```python
from build123d import *

# Parameters (mm, degrees)
SALIENTE_EXTRUIR2_DEPTH      = 69
SALIENTE_EXTRUIR2_DEPTH_BACK = 69
CROQUIS3_R                   = 58
CROQUIS5_R                   = 58
CROQUIS5_R_2                 = 47.65301306
CROQUIS5_R_3                 = 3.895689101
SALIENTE_EXTRUIR3_DEPTH      = 2


with BuildPart() as part:
    # Croquis2 → Revolución1 (revolve)
    with BuildSketch(Plane.XY):
        Polygon((0, 0), (-58, 0), (-58, 68), (-42.5, 83.579391827), (-42.5, 378.579391827), (-58, 394.000404577), (-58, 462.000404577), (0, 462.000404577), align=None)
    revolve(axis=Axis((0, 462.000404577, 0), (0, -1, 0)))

    # Croquis3 → Saliente-Extruir2 (add, two sides: drawn at the far end of the back side and taken through both)
    with BuildSketch(Plane(origin=(0, 0, 0), x_dir=(0, 0, -1), z_dir=(1, 0, 0)).offset(-SALIENTE_EXTRUIR2_DEPTH_BACK)):
        with Locations((0, 462.000404577)):
            Circle(CROQUIS3_R)
        Circle(CROQUIS3_R)
    extrude(amount=SALIENTE_EXTRUIR2_DEPTH + SALIENTE_EXTRUIR2_DEPTH_BACK)

    # Croquis5 → Saliente-Extruir3 (add)
    # profile 1 of 2: a face of its own
    with BuildSketch(Plane(origin=(69, 0, 0), x_dir=(0, 0, -1), z_dir=(1, 0, 0))):
        Circle(CROQUIS5_R)
        Circle(CROQUIS5_R_2, mode=Mode.SUBTRACT)
        with Locations((0, 52.526315759)):
            Circle(CROQUIS5_R_3, mode=Mode.SUBTRACT)
        with Locations((49.95549488, 16.231524222)):
            Circle(CROQUIS5_R_3, mode=Mode.SUBTRACT)
        with Locations((30.874193761, -42.494682101)):
            Circle(CROQUIS5_R_3, mode=Mode.SUBTRACT)
        with Locations((-30.874193761, -42.494682101)):
            Circle(CROQUIS5_R_3, mode=Mode.SUBTRACT)
        with Locations((-49.95549488, 16.231524222)):
            Circle(CROQUIS5_R_3, mode=Mode.SUBTRACT)
    # profile 2 of 2: a face of its own
    with BuildSketch(Plane(origin=(69, 0, 0), x_dir=(0, 0, -1), z_dir=(1, 0, 0))):
        with Locations((0, 462.000404577)):
            Circle(CROQUIS5_R)
        with Locations((0, 462.000404577)):
            Circle(CROQUIS5_R_2, mode=Mode.SUBTRACT)
        with Locations((-49.95549488, 478.231928798)):
            Circle(CROQUIS5_R_3, mode=Mode.SUBTRACT)
        with Locations((0, 514.526720336)):
            Circle(CROQUIS5_R_3, mode=Mode.SUBTRACT)
        with Locations((30.874193761, 419.505722476)):
            Circle(CROQUIS5_R_3, mode=Mode.SUBTRACT)
        with Locations((-30.874193761, 419.505722476)):
            Circle(CROQUIS5_R_3, mode=Mode.SUBTRACT)
        with Locations((49.95549488, 476.231524222)):
            Circle(CROQUIS5_R_3, mode=Mode.SUBTRACT)
    extrude(amount=SALIENTE_EXTRUIR3_DEPTH)


solid = part.part
```
The listing builds one solid part. Answer for the finished solid, in the listing's coordinates (mm). A direction names the side the tool comes from. Give positions to 0.01 mm unless a question says otherwise; leave off trailing zeros. Order: outer loops, then holes, each group sorted by start corner. A loop starts at its lowest first (then second) coordinate and runs counter-clockwise, first axis right, second up. Notation, with made-up numbers: (32.25, -40) -> (43.25, -40) arc R17 ccw to (43.25, -28) -> close; hole circle Ø1 at (21, -27). An arc over 180 degrees is marked (long way). One line per item, written item: value.
1) Find section B-B, the plane y = 100. Determine the outline of the cut face in (x, z).
Reported:
outline: circle Ø85 at (0, 0)
2) Flat-ended cylindrical pins translate along their axes: P1, Ø5, axis at x = 3.5, z = -32, coming from the +Y side; P2, Ø6, axis at y = 476.23, z = -49.96, coming from the +X side; P3, Ø3, axis at y = 183, z = 13, coming from the +X side. Find the tip coordinate at first contact, or state that the pin passes through.
Reported:
P1: stops at y = 511.94
P2: stops at x = 69
P3: stops at x = 40.91
3) Find section A-A, the plane x = 0. Determine the outline of the cut face in (y, z), plus the area to 3 significant figures.
Reported:
outline: (0, -58) -> (68, -58) -> (83.58, -42.5) -> (378.58, -42.5) -> (394, -58) -> (462, -58) arc R58 ccw to (462, 58) -> (394, 58) -> (378.58, 42.5) -> (83.58, 42.5) -> (68, 58) -> (0, 58) arc R58 ccw to start
area: 54,500 mm^2
4) Determine the mould class of faces 1 (the cylindrical face through (69.986, -28.996, 37.816)), 2 (the flat face through (-69, 1, 1)), 3 (the conical face through (5.631, 82.823, -42.885)) for opening direction Z: pulls with the +Z half, pulls with the -Z half, needs draft (parallel to the pull), parting line crosses it, or undercut.
Reported:
face 1: undercut
face 2: needs draft
face 3: parting line crosses it
5) Find the intervals of material crossed by line 1 (Y direction, x = 69.55, z = 0); line 2 (X direction, y = 441, z = -21); line 3 (Z direction, x = -3, y = 210.5), in increasing order.
Reported:
line 1: y = -58 to -47.65, 47.65 to 48.63, 56.42 to 58, 404 to 414.35, 509.65 to 510.63, 518.42 to 520
line 2: x = -69 to 69
line 3: z = -42.39 to 42.39
6) A tool of negligible diameter and unlimited length cuts with its end or side. For faces 4 (the conical face through (-20.059, 379.544, 38.565)), 5 (the flat face through (69, 1, 1)), 6 (the flat face through (71, 48, -4)), from which of +Z, -Z, +X, -X, +Y, -Y can it reach the whole face along a straight path? Write none if from no direction.
Reported:
face 4: none
face 5: +X
face 6: +Z, -Z, +X, +Y, -Y
